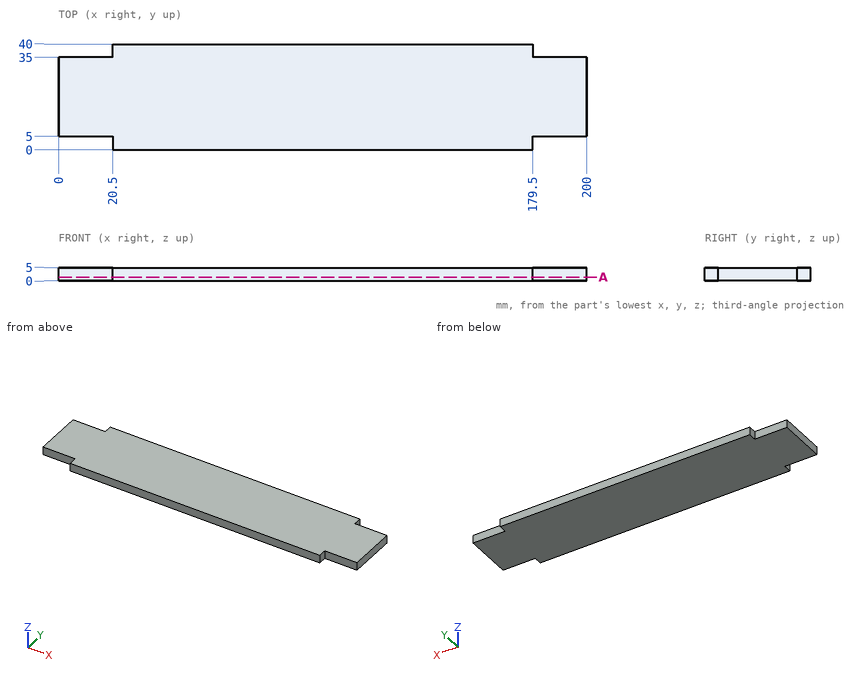
Design review of the part shown in the three views and the two pictorial views. Dimensions are in mm from the part's minimum x, y and z. Give positions to 0.01 mm unless a question says otherwise; leave off trailing zeros. Write each loop counter-clockwise with the first axis right and the second up, starting at its lowest first coordinate (ties: lowest second). Pieces come first, ordered by that corner, then holes. Notation, with made-up numbers: M 69,-4 L 76,-4 A8 cw 76,6 Z; hole C -21.75,-3 d7. An arc over 180 degrees is marked long. Return JSON: item names as keys, results as strings. Group by question number.
Item 1: Take a section at A-A (z = 1.45). Give the boundary of the cut face in (x, y), plus the area to 3 significant figures.
Item 2: Wall thickness on line 1 along X through (y, z) = (36, 4.35); line 2 along Y through (x, z) = (10, 1.1): over which ranges is each line inside the solid? List them lowest first.
Item 3: Clearance check with flat-ended pins moving along their axes: pin 1 Ø2.5 at (y, z) = (3, 1.5) entering from +X; pin 2 Ø2.5 at (x, z) = (7.5, 3.5) entering from +Y; pin 3 Ø1.5 at (y, z) = (3.5, 1.5) entering from -X. State where each tip first meets the part, or that it passes through.
Return value:
{
 "1": {"outline": "M 0,5 L 20.5,5 L 20.5,0 L 179.5,0 L 179.5,5 L 200,5 L 200,35 L 179.5,35 L 179.5,40 L 20.5,40 L 20.5,35 L 0,35 Z", "area": "7,590 mm2"},
 "2": {"line 1": "x = 20.5 to 179.5", "line 2": "y = 5 to 35"},
 "3": {"pin 1": "stops at x = 179.5", "pin 2": "stops at y = 35", "pin 3": "stops at x = 20.5"}
}
